Verification items for the finished model (mm, model axes). Face numbers are marked on the shaded views. A direction names the side the tool comes from. Coordinates: 2 decimals unless noted, no trailing zeros. Order: outer loops, then holes, each group sorted by start corner. A loop starts at its lowest first (then second) coordinate and runs counter-clockwise, first axis right, second up. Notation, with made-up numbers: M 74.5,74 L 112.5,74 A23 ccw 112.5,88 Z; hole C -21.75,-21.5 d11. An arc over 180 degrees is marked long. Return JSON: item names as keys, results as strings. Group by question number.
Q1. Section check C-C, the plane z = 3.75. Enter the section's corners in (x, y), then the cut area to 3 significant figures.
Q2. Go/stop test with flat-tipped pins: pin 1 Ø1 at (x, z) = (3.5, 6) entering from +Y; pin 2 Ø0.9 at (y, z) = (1, 4) entering from -X. Record where each tip stops, or that it passes through.
Q3. Section check D-D, the plane y = 0.3. Enter the section's corners in (x, z).
Q4. Access from +Z, -Z, +X, -X, +Y, -Y to the whole of each face (thin tool, end or side, straight path). Record for the marked faces 1 and 2.
Q5. Section check A-A, the plane x = 3.5. Enter the section's corners in (y, z).
Q6. Section check B-B, the plane y = -1.6. Enter the section's corners in (x, z).
Q7. Thickness scan on probe 1 along Y at (x, z) = (1, 3.75); probe 2 along X at (y, z) = (0.05, 3.75); probe 3 along Z at (x, y) = (5.5, 1.6). Record the ranges inside material, lowest first.
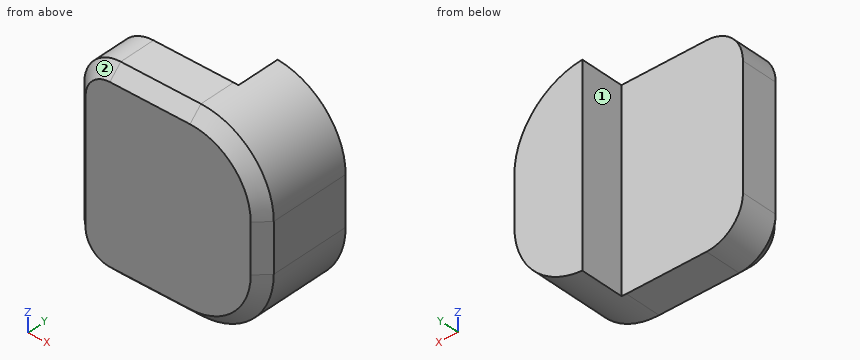
from build123d import *

# Parameters (mm, degrees)
BOSS_EXTRUDE1_DEPTH = 8
FILLET1_R           = 3
FILLET2_R           = 1.5
CHAMFER1_SIZE       = 0.5


with BuildPart() as part:
    # Sketch1 → Boss-Extrude1 (new body)
    with BuildSketch(Plane.XY):
        Polygon((0, 0), (5, 0), (5, 1.8), (7.8, 1.8), (7.8, 0), (7.8, -0.329113924), (7.8, -2), (6.430379747, -2), (0, -2), align=None)
    extrude(amount=BOSS_EXTRUDE1_DEPTH)

    # Fillet1
    fillet1_edges = [part.edges().sort_by_distance(p)[0] for p in [
        (7.8, -0.1, 0),
        (7.8, -0.1, 8),
    ]]
    fillet(fillet1_edges, radius=FILLET1_R)

    # Fillet2
    fillet2_edges = [part.edges().sort_by_distance(p)[0] for p in [
        (0, -1, 0),
        (0, -1, 8),
    ]]
    fillet(fillet2_edges, radius=FILLET2_R)

    # Chamfer1
    chamfer1_edges = [part.edges().sort_by_distance(p)[0] for p in [
        (7.8, -2, 4),
        (6.921320344, -2, 7.121320344),
        (6.921320344, -2, 0.878679656),
        (0, -2, 4),
        (3.15, -2, 0),
        (3.15, -2, 8),
        (0.439339828, -2, 7.560660172),
        (0.439339828, -2, 0.439339828),
    ]]
    chamfer(chamfer1_edges, length=CHAMFER1_SIZE)


solid = part.part
Numbers:
{
 "1": {"outline": "M 0,-1.5 L 0.5,-2 L 7.3,-2 L 7.8,-1.5 L 7.8,1.8 L 5,1.8 L 5,0 L 0,0 Z", "area": "20.4 mm2"},
 "2": {"pin 1": "stops at y = 0", "pin 2": "stops at x = 5"},
 "3": {"outline": "M 5,0.01 A3 ccw 7.8,3 L 7.8,5 A3 ccw 5,7.99 Z"},
 "4": {"face 1": "+Z, -Z, -X, +Y", "face 2": "+Z, -X, -Y"},
 "5": {"outline": "M -2,0.5 L -1.5,0 L 0,0 L 0,8 L -1.5,8 L -2,7.5 Z"},
 "6": {"outline": "M 0.1,1.5 A1.4 ccw 1.5,0.1 L 4.8,0.1 A2.9 ccw 7.7,3 L 7.7,5 A2.9 ccw 4.8,7.9 L 1.5,7.9 A1.4 ccw 0.1,6.5 Z"},
 "7": {"probe 1": "y = -2 to 0", "probe 2": "x = 5 to 7.8", "probe 3": "z = 0.08 to 7.92"}
}
